```python
from build123d import *

# Parameters (mm, degrees)
BOSS_EXTRUDE1_DEPTH = 0.9
FILLET1_R           = 0.5
BOSS_EXTRUDE2_DEPTH = 10
BOSS_EXTRUDE3_DEPTH = 10
BOSS_EXTRUDE4_DEPTH = 10
CUT_EXTRUDE2_DEPTH  = 61.26562122547703
FILLET2_R           = 10
CUT_EXTRUDE3_DEPTH  = 61.26562122547703
CUT_EXTRUDE4_DEPTH  = 61.265621208883815
FILLET3_R           = 0.6
SKETCH10_R          = 2.1
BOSS_EXTRUDE5_DEPTH = 3
SKETCH11_R          = 1.5
BOSS_EXTRUDE6_DEPTH = 2
BOSS_EXTRUDE7_DEPTH = 3
SKETCH14_R          = 1.5000000000000002
BOSS_EXTRUDE8_DEPTH = 2
FILLET4_R           = 0.5


# Read off the part's stored shape, not the designer's step: Split1
with BuildPart() as part:
    # Sketch1 → Boss-Extrude1 (new body)
    with BuildSketch(Plane(origin=(0, 0, 0), x_dir=(0, 0, -1), z_dir=(1, 0, 0))):
        with BuildLine():
            Line((0, 2.8), (0, 0))
            add(Edge.make_bspline(
                [(0, 0), (-5.0882686653691644, 0), (-6.101472647573343, 1.7391212131518174), (-7.000000000000001, 5.128421052631583)],
                knots=[0, 0, 0, 0, 1, 1, 1, 1], degree=3))
            add(Edge.make_bspline(
                [(-7.000000000000001, 5.128421052631583), (-4.554183023047009, 3.433770739772326), (-3.654213934684202, 2.799999999999996), (0, 2.8)],
                knots=[0, 0, 0, 0, 1, 1, 1, 1], degree=3))
        make_face()
    extrude(amount=BOSS_EXTRUDE1_DEPTH)

    # Fillet1
    fillet1_edges = [part.edges().sort_by_distance(p)[0] for p in [
        (0.45, 5.128421052631583, 7.000000000000001),
    ]]
    fillet(fillet1_edges, radius=FILLET1_R)

    # Sketch3 → Boss-Extrude2 (add)
    with BuildSketch(Plane(origin=(0, 0, 0), x_dir=(0, 0, -1), z_dir=(1, 0, 0))):
        Polygon((0, 0), (40, 0), (40, 10), (20, 9.999999999999998), (0, 2.8), align=None)
    extrude(amount=BOSS_EXTRUDE2_DEPTH)

    # Sketch5 → Boss-Extrude3 (add)
    with BuildSketch(Plane(origin=(0, 0, 0), x_dir=(0, 0, -1), z_dir=(1, 0, 0))):
        Polygon((0, 0), (20.000000000000004, -11.54700538379255), (40, -11.547005383792548), (40, 0), align=None)
    extrude(amount=BOSS_EXTRUDE3_DEPTH)

    # Sketch6 → Boss-Extrude4 (add)
    with BuildSketch(Plane(origin=(10, 0, 0), x_dir=(0, 0, -1), z_dir=(1, 0, 0))):
        Polygon((8.351482323931023, -4.821730567853972), (55.39585291736738, 12.114242845783108), (52.00865823463995, 21.523116964470375), (20, 9.999999999999998), align=None)
    extrude(amount=-BOSS_EXTRUDE4_DEPTH)

    # Sketch7 → Cut-Extrude2 (cut, through all)
    with BuildSketch(Plane(origin=(10, 0, 0), x_dir=(0, 0, -1), z_dir=(1, 0, 0))):
        Polygon((40, 6.571735795530855), (-6.396657859934056, -10.1310610340454), (25.03138273349842, -20.31963634568749), (52.56184703999606, -5.85197020171655), align=None)
    extrude(amount=-CUT_EXTRUDE2_DEPTH, mode=Mode.SUBTRACT)

    # Fillet2
    fillet2_edges = [part.edges().sort_by_distance(p)[0] for p in [
        (5, -4.821730567853985, -8.351482323931002),
    ]]
    fillet(fillet2_edges, radius=FILLET2_R)

    # Sketch8 → Cut-Extrude3 (cut, through all)
    with BuildSketch(Plane(origin=(10, 0, 0), x_dir=(0, 0, -1), z_dir=(1, 0, 0))):
        with BuildLine():
            Line((2, 1.15470053837925), (5.3316294573154766, -0.7688166256419326))
            ThreePointArc((5.3316294573154766, -0.7688166256419326), (8.6203969477251, -1.8089349449339256), (12.041385203497414, -1.3677126903162435))
            Line((12.041385203497414, -1.3677126903162435), (52.83663915708444, 13.318578732975077))
            Line((52.83663915708444, 13.318578732975077), (50.80432234744798, 18.963903204187442))
            Line((50.80432234744798, 18.963903204187442), (2, 1.394347159106174))
            Line((2, 1.394347159106174), (2, 1.15470053837925))
        make_face()
    extrude(amount=-CUT_EXTRUDE3_DEPTH, mode=Mode.SUBTRACT)

    # Sketch9 → Cut-Extrude4 (cut, through all)
    with BuildSketch(Plane.ZY):
        Polygon((3.0000000000000013, -0.988739395943905), (3.0000000000000004, 5.799008427986812), (9.091562908025708, 5.799008427986812), (9.091562908025708, -1.8536705996620422), align=None)
    extrude(amount=-CUT_EXTRUDE4_DEPTH, mode=Mode.SUBTRACT)

    # Fillet3
    fillet3_edges = [part.edges().sort_by_distance(p)[0] for p in [
        (0.45, 0.2958164494648414, 3.0000000000000013),
        (0.45, 3.0492242349736607, 3.000000000000001),
    ]]
    fillet(fillet3_edges, radius=FILLET3_R)

    # Sketch10 → Boss-Extrude5 (add)
    with BuildSketch(Plane(origin=(0, 19.04436342339395, -52.90100950942748), x_dir=(-1, 0, 0), z_dir=(0, 0.33871946827274263, -0.9408874118687265))):
        with Locations(Location((-5, -2.365515246767623, 0), (0, 0, 270))):
            Circle(SKETCH10_R)
    extrude(amount=BOSS_EXTRUDE5_DEPTH)

    # Sketch11 → Boss-Extrude6 (add)
    with BuildSketch(Plane(origin=(0, 20.060521828212188, -55.72367174503367), x_dir=(-1, 0, 0), z_dir=(0, 0.33871946827274263, -0.9408874118687265))):
        with Locations(Location((-5, -2.365515246767633, 0), (0, 0, 90))):
            Circle(SKETCH11_R)
    extrude(amount=BOSS_EXTRUDE6_DEPTH)


with BuildPart() as body_2:
    # Split1: the piece on the far side of the plane
    add(part.part)
    split(bisect_by=Plane(origin=(0, 19.044363423, -52.901009509), x_dir=(1, 0, 0), z_dir=(0, 0.33871946827274285, -0.9408874118687265)), keep=Keep.BOTTOM)


with BuildPart() as part_1:
    add(part.part)

    # Split1
    split(bisect_by=Plane(origin=(0, 19.044363423, -52.901009509), x_dir=(1, 0, 0), z_dir=(0, 0.33871946827274285, -0.9408874118687265)), keep=Keep.TOP)


with BuildPart() as body_3:
    # Sketch13 → Boss-Extrude7 (new body)
    with BuildSketch(Plane(origin=(0, 19.04436342339395, -52.90100950942748), x_dir=(-1, 0, 0), z_dir=(0, 0.33871946827274263, -0.9408874118687265))):
        Polygon((-3.4648232278140823, -4.097926860674667), (6e-17, -4.097926860674667), (4e-17, -0.6331036328605839), (-3.4648232278140823, -0.6331036328605846), align=None)
    extrude(amount=BOSS_EXTRUDE7_DEPTH)


with BuildPart() as body_4:
    # Sketch14 → Boss-Extrude8 (new body)
    with BuildSketch(Plane(origin=(0, 20.060521828212188, -55.72367174503367), x_dir=(-1, 0, 0), z_dir=(0, 0.33871946827274263, -0.9408874118687265))):
        with Locations(Location((-1.7324116139070413, -2.3655152467676324, 0), (0, 0, 90))):
            Circle(SKETCH14_R)
    extrude(amount=BOSS_EXTRUDE8_DEPTH)


with BuildPart() as body_2_1:
    add(body_2.part)

    # Combine1: union body 3, body 4
    add(body_3.part)
    add(body_4.part)

    # Fillet4
    fillet4_edges = [body_2_1.edges().sort_by_distance(p)[0] for p in [
        (-6e-17, 15.69675482783554, -55.70038823449888),
        (-4e-17, 18.95676338723618, -54.526785153114645),
        (3.4648232278140823, 18.95676338723618, -54.526785153114645),
        (3.4648232278140823, 15.69675482783554, -55.70038823449888),
    ]]
    fillet(fillet4_edges, radius=FILLET4_R)


solid = body_2_1.part
```
Source: CAD feature listing. Evaluate the final solid. Frame: model axes, mm. A direction names the side the tool comes from. Coordinates: 2 decimals unless noted, no trailing zeros. Loops run counter-clockwise (first coordinate to the right, second up) from the corner with the lowest first, then second, coordinate; pieces in that order, holes last. Notation, with made-up numbers: M 25.5,-4.75 L 59.5,-4.75 A25 ccw 59.5,21.25 Z; hole C 86.5,60 d11. An arc over 180 degrees is marked long. Use a Markdown table: item, result. Add a question column.
Q1. Material intervals for L1, parallel to Y at x = 2.5, z = -26; L2, parallel to Y at x = 2.75, z = -9, sorted ascending.
Q2. Access query for faces 1 (the flat face through (1.75, 15.69, -55.68)), 2 (the flat face through (5, 1, 0)), 3 (the cylindrical face through (3.314, 15.838, -55.672)), 4 (the flat face through (5, 0, -4)), 5 (the flat face through (3.465, 17, -55)). Directions: +Z, -Z, +X, -X, +Y, -Y. A direction counts if a zero-diameter tool reaches every point of the face in a straight line with its end or side. Return the directions, or none.
Q3. Section query B-B, the plane x = 9. Return loops of the section in (y, z), and give its area (3 significant figures).
Q4. Draft query along Y for faces 6 (the cylindrical face through (3.31, 18.83, -54.59)), 7 (the flat face through (0, 12, -29)), 8 (the flat face through (5.07, 5.87, -32.15)), 9 (the flat face through (5.07, 16.102, -51.835)). Return one class per face: pulls with the +Y half, pulls with the -Y half, needs draft (parallel to the pull), parting line crosses it, or undercut.
Q5. First-contact query: pin 1 (5 mm diameter, centred on x = 3, z = -3.5, fed in from +Y); pin 2 (1.7 mm diameter, centred on y = 17.5, z = -54.5, fed in from +X); pin 3 (5 mm diameter, centred on x = 3.5, z = -9, fed in from +Y). Flat tips, straight axial feed; report the tip coordinate or a pass-through.
Q6. Section query C-C, the plane z = -43. Return loops of the section in (x, y), and give its area (3 significant figures).
Q7. Section query A-A, the plane y = 14.5. Return loops of the section in (x, z), and give its area (3 significant figures).
Result:
| question | item | result |
|---|---|---|
| 1 | L1 | y = 1.53 to 3.66, 10.03 to 12.16 |
| 1 | L2 | y = -3.84 to -1.83, 3.91 to 6.04 |
| 2 | face 1 | -Z, +X, -X |
| 2 | face 2 | +Z, +X, +Y, -Y |
| 2 | face 3 | -Z, +X |
| 2 | face 4 | +X, -X |
| 2 | face 5 | -Z, +X, +Y |
| 3 | outline | M -3.25,-12.72 L 12.11,-55.4 L 21.52,-52.01 L 2.8,0 L 0,0 L -2.5,-4.33 A10 ccw Z; hole M -1.37,-12.04 L 13.32,-52.84 L 18.96,-50.8 L 1.39,-2 L 1.15,-2 L -0.77,-5.33 A8 ccw Z |
| 3 | area | 239 mm2 |
| 4 | face 6 | pulls with the +Y half |
| 4 | face 7 | needs draft |
| 4 | face 8 | undercut |
| 4 | face 9 | undercut |
| 5 | pin 1 | stops at y = 4.96 |
| 5 | pin 2 | stops at x = 3.46 |
| 5 | pin 3 | stops at y = 6.94 |
| 6 | outline | M 0,7.65 L 10,7.65 L 10,9.78 L 0,9.78 Z; M 0,16.15 L 10,16.15 L 10,18.28 L 0,18.28 Z |
| 6 | area | 42.5 mm2 |
| 7 | outline | M 0,-54.54 L 10,-54.54 L 10,-52.41 L 0,-52.41 Z; M 0,-38.4 L 10,-38.4 L 10,-32.5 L 0,-32.5 Z |
| 7 | area | 80.3 mm2 |
